The listing builds one solid part. Answer for the finished solid, in the listing's coordinates (mm). A direction names the side the tool comes from. Round coordinates to 2 decimals unless told otherwise and drop trailing zeros. Write each loop counter-clockwise with the first axis right and the second up, starting at its lowest first coordinate (ties: lowest second). Pieces come first, ordered by that corner, then holes. Notation, with made-up numbers: (65, 41.25) - (89, 41.25) arc R28 cw to (89, 59.25) - close; hole circle Ø4 at (13.25, -17). An arc over 180 degrees is marked (long way). Use a Markdown table: item, result. Add a question column.
1) A cutting plane is placed at B-B (y = 4). Give the vertices of the cut face in (x, z), then the cut area to 3 significant figures.
2) A cutting plane is placed at C-C (x = -5.5). Give the vertices of the cut face in (y, z).
3) A tool of negligible diameter and unlimited length cuts with its end or side. For faces 5 (the cylindrical face through (-7.63, -16.31, 12.89)), 6 (the flat face through (2, 10.199, 7)), 7 (the flat face through (0.1, 11.699, 3.2)), from which of +Z, -Z, +X, -X, +Y, -Y can it reach the whole face along a straight path? Write none if from no direction.
4) Determine the mould class of faces 1 (the cylindrical face through (10.9, 7.8, 6.6)), 2 (the flat face through (0, 16.699, 10)), 3 (the cylindrical face through (-4.27, 15.96, 8.14)), 4 (the flat face through (-4, 15.199, 8)) for opening direction Y: +Y half, -Y half, draft (parallel to the pull), parting line (faces both ways), or undercut.
5) A cutting plane is placed at D-D (x = 7.75). Give the vertices of the cut face in (y, z), then the cut area to 3 significant figures.
6) Each of these flat-tipped pins is pushed along its axis until it touches: P1, Ø0.8, axis at x = 0, y = 11, coming from the -Z side; P2, Ø1.6, axis at y = 11, z = 1.5, coming from the +X side; P3, Ø4, axis at y = 0.5, z = 4.5, coming from the +X side. Where does it stop, or does it pass through?
7) A cutting plane is placed at A-A (x = 4). Give the vertices of the cut face in (y, z).
8) Find the intervals of material crossed by probe 1 along Y at (x, z) = (-8.25, 3.5); probe 2 along Z at (x, y) = (-7.5, -16.3); probe 3 along Y at (x, z) = (-6.5, 10.25), in increasing order. Write a range as from..to.
```python
from build123d import *

# Parameters (mm, degrees)
F1_DEPTH  = 4.5
F3_DEPTH  = 10.4
F5_DEPTH  = 13.4
F6_R      = 3.7
F6_R_2    = 1.6
F7_DEPTH  = 5
F8_R      = 1.6
F8_R_2    = 3.7
F9_DEPTH  = 5
F10_R     = 1
F11_DEPTH = 2
F12_W     = 10
F12_H     = 1.5
F13_DEPTH = 3


with BuildPart() as f1:
    # F0 (on Top) → F1 (new body)
    with BuildSketch(Plane.XY):
        with BuildLine():
            ThreePointArc((-14, -13.8007847667), (-12.9748737342, -16.2756585008), (-10.5, -17.3007847667))
            Line((-10.5, -17.3007847667), (-6.75, -17.3007847667))
            Line((-6.75, -17.3007847667), (6.75, -17.3007847667))
            Line((6.75, -17.3007847667), (10.5, -17.3007847667))
            ThreePointArc((10.5, -17.3007847667), (12.9748737342, -16.2756585008), (14, -13.8007847667))
            Line((14, -13.8007847667), (14, -11.8007847667))
            Line((14, -11.8007847667), (13.0486556537, 6.7504299853))
            ThreePointArc((13.0486556537, 6.7504299853), (11.6774697173, 9.4001806183), (9.7759521317, 11.6992152333))
            Line((9.7759521317, 11.6992152333), (-9.7759521317, 11.6992152333))
            ThreePointArc((-9.7759521317, 11.6992152333), (-11.6774697173, 9.4001806183), (-13.0486556537, 6.7504299853))
            Line((-13.0486556537, 6.7504299853), (-14, -11.8007847667))
            Line((-14, -11.8007847667), (-14, -13.8007847667))
        make_face()
    extrude(amount=F1_DEPTH)

    # F2 (on face) → F3 (join)
    with BuildSketch(Plane.XY.offset(4.5)):
        with BuildLine():
            Line((14, -13.8007847667), (14, -11.8007847667))
            Line((14, -11.8007847667), (13.0486556537, 6.7504299853))
            add(Edge.make_bspline(
                [(13.0486556537, 6.7504299853), (12.8450421616, 12.0132155716), (11.5178218111, 15.1653625071), (9.2356767608, 16.6992152333)],
                knots=[0, 0, 0, 0, 10.6544420759, 10.6544420759, 10.6544420759, 10.6544420759], degree=3))
            Line((9.2356767608, 16.6992152333), (-9.2356767608, 16.6992152333))
            add(Edge.make_bspline(
                [(-13.0486556537, 6.7504299853), (-12.8450421616, 12.0132155716), (-11.5178218111, 15.1653625071), (-9.2356767608, 16.6992152333)],
                knots=[0, 0, 0, 0, 10.6544420759, 10.6544420759, 10.6544420759, 10.6544420759], degree=3))
            Line((-13.0486556537, 6.7504299853), (-14, -11.8007847667))
            Line((-14, -11.8007847667), (-14, -13.8007847667))
            ThreePointArc((-14, -13.8007847667), (-12.9748737342, -16.2756585008), (-10.5, -17.3007847667))
            Line((-10.5, -17.3007847667), (10.5, -17.3007847667))
            ThreePointArc((10.5, -17.3007847667), (12.9748737342, -16.2756585008), (14, -13.8007847667))
        make_face()
    extrude(amount=F3_DEPTH)

    # F4 (on face) → F5 (cut)
    with BuildSketch(Plane.XY):
        with BuildLine():
            Line((0, -15.3007847667), (8.5, -15.3007847667))
            ThreePointArc((8.5, -15.3007847667), (10.9748737342, -14.2756585008), (12, -11.8007847667))
            Line((12, -11.8007847667), (12, 5.1777003818))
            ThreePointArc((12, 5.1777003818), (10.8666119051, 7.8556244429), (9.145150881, 10.1992152333))
            Line((9.145150881, 10.1992152333), (-9.145150881, 10.1992152333))
            ThreePointArc((-9.145150881, 10.1992152333), (-10.8666119051, 7.8556244429), (-12, 5.1777003818))
            Line((-12, 5.1777003818), (-12, -11.8007847667))
            ThreePointArc((-12, -11.8007847667), (-10.9748737342, -14.2756585008), (-8.5, -15.3007847667))
            Line((-8.5, -15.3007847667), (0, -15.3007847667))
        make_face()
    extrude(amount=F5_DEPTH, mode=Mode.SUBTRACT)

    # F6 (on face) → F7 (cut)
    with BuildSketch(Plane(origin=(0, 16.6992152333, 0), x_dir=(-1, 0, 0), z_dir=(0, 1, 0))):
        with Locations((-4.6178383804, 9.7)):
            Circle(F6_R)
        with Locations((4.6178383804, 9.7)):
            Circle(F6_R_2)
    extrude(amount=-F7_DEPTH, mode=Mode.SUBTRACT)

    # F8 (on face) → F9 (cut)
    with BuildSketch(Plane.XZ.offset(-10.1992152333)):
        with Locations((4.6178383804, 9.7)):
            Circle(F8_R)
        with Locations((-4.6178383804, 9.7)):
            Circle(F8_R_2)
    extrude(amount=-F9_DEPTH, mode=Mode.SUBTRACT)

    # F10 (on face) → F11 (cut, through all)
    with BuildSketch(Plane.XZ.offset(17.3007847667)):
        with Locations((-7.5, 11.9)):
            Circle(F10_R)
    extrude(amount=-F11_DEPTH, mode=Mode.SUBTRACT)

    # F12 (on face) → F13 (cut)
    with BuildSketch(Plane(origin=(0, 0, 0), x_dir=(1, 0, 0), z_dir=(0, 0, -1))):
        with Locations((0, -10.9492152333)):
            Rectangle(F12_W, F12_H)
    extrude(amount=-F13_DEPTH, mode=Mode.SUBTRACT)


solid = f1.part
```
Entries:
| question | item | result |
|---|---|---|
| 1 | outline | (-13.19, 0) - (-12, 0) - (-12, 13.4) - (12, 13.4) - (12, 0) - (13.19, 0) - (13.19, 14.9) - (-13.19, 14.9) - close |
| 1 | area | 71.5 mm² |
| 2 | outline | (-17.3, 0) - (-15.3, 0) - (-15.3, 13.4) - (10.2, 13.4) - (10.2, 13.29) - (15.2, 13.29) - (15.2, 11.03) - (16.7, 11.03) - (16.7, 14.9) - (-17.3, 14.9) - close; (10.2, 0) - (11.7, 0) - (11.7, 4.5) - (16.7, 4.5) - (16.7, 8.37) - (15.2, 8.37) - (15.2, 6.11) - (10.2, 6.11) - close |
| 3 | face 5 | -Y |
| 3 | face 6 | -Z |
| 3 | face 7 | -Z, +X, -X, +Y |
| 4 | face 1 | undercut |
| 4 | face 2 | +Y half |
| 4 | face 3 | draft |
| 4 | face 4 | undercut |
| 5 | outline | (-17.3, 0) - (-15.3, 0) - (-15.3, 13.4) - (10.2, 13.4) - (10.2, 0) - (11.7, 0) - (11.7, 4.5) - (16.7, 4.5) - (16.7, 7.73) - (11.7, 7.73) - (11.7, 11.67) - (16.7, 11.67) - (16.7, 14.9) - (-17.3, 14.9) - close |
| 5 | area | 123 mm² |
| 6 | P1 | stops at z = 3 |
| 6 | P2 | stops at x = 11.11 |
| 6 | P3 | stops at x = 13.47 |
| 7 | outline | (-17.3, 0) - (-15.3, 0) - (-15.3, 13.4) - (10.2, 13.4) - (10.2, 11.18) - (11.7, 11.18) - (11.7, 13.35) - (16.7, 13.35) - (16.7, 14.9) - (-17.3, 14.9) - close; (10.2, 3) - (11.7, 3) - (11.7, 4.5) - (16.7, 4.5) - (16.7, 6.05) - (11.7, 6.05) - (11.7, 8.22) - (10.2, 8.22) - close |
| 8 | probe 1 | y = -17.3..-15.3, 10.2..11.7 |
| 8 | probe 2 | z = 0..10.9, 12.9..14.9 |
| 8 | probe 3 | y = -17.3..-15.3, 15.2..16.7 |
